Source: CAD feature listing. Evaluate the final solid. Frame: model axes, mm. A direction names the side the tool comes from. Give positions to 0.01 mm unless a question says otherwise; leave off trailing zeros. Order: outer loops, then holes, each group sorted by start corner. A loop starts at its lowest first (then second) coordinate and runs counter-clockwise, first axis right, second up. Notation, with made-up numbers: M 83,88.5 L 118,88.5 A12 ccw 118,101.5 Z; hole C 50.5,47.25 d10. An arc over 180 degrees is marked long. Use CSV: the item, a comma, the result in double quotes. Start each with the question number.
1. Pin query (flat end, axial travel): P1, Ø6, axis at x = 78, z = 2.5, coming from the +Y side; P2, Ø3, axis at x = -69, y = 5, coming from the +Z side; P3, Ø2, axis at x = 55.5, y = 2, coming from the +Z side. Return the tip coordinate at first contact, or that it passes through.
2. Section query A-A, the plane x = 77.5. Return the cut outline in (y, z), plus the area to 3 significant figures.
3. Line query: line 1 along Z through (x, y) = (65, 3.5); line 2 along X through (y, z) = (1.5, 4); line 3 along X through (y, z) = (1.5, -13.5). Output: solid intervals per line, ascending. Write a range as [from, to].
4. Section query B-B, the plane z = -67.5. Return the cut outline in (x, y).
5. Section query C-C, the plane y = 2. State how many separate pieces and enclosed holes the cut face has, plus the area to 3 significant figures.
6. Reachability of faces 5 (the flat face through (4, 10, -1)), 6 (the flat face through (33.887, 5, 8)), 7 (the flat face through (-80.901, 5, -85)), 8 (the cylindrical face through (76.395, 7.535, -7.936)), 9 (the flat face through (-80.901, 5, 85)) from +Z, -Z, +X, -X, +Y, -Y: full face, straight path, thin tool, end or side. Return the list, or none.
7. Mould query, pull axis Z, two halves, no side actions, for faces 1 (the flat face through (-65, 5, -80)), 2 (the flat face through (33.887, 5, -8)), 3 (the flat face through (-85, 5, 90)), 4 (the cylindrical face through (-43.254, 4.93, 88.662)). Classes: released by +Z, released by -Z, zero draft, split by the parting line, or undercut.
8. Section query D-D, the plane x = -72.5. Return the cut outline in (y, z), plus the area to 3 significant figures.
from build123d import *

# Parameters (mm, degrees)
BOSS_EXTRUDE1_DEPTH = 10
SKETCH2_R           = 1
SKETCH2_R_2         = 1.5
SKETCH2_W           = 33
SKETCH2_H           = 10
CUT_EXTRUDE2_DEPTH  = 15
SKETCH3_R           = 10
CUT_EXTRUDE3_DEPTH  = 5


with BuildPart() as part:
    # Sketch1 → Boss-Extrude1 (new body)
    with BuildSketch(Plane(origin=(0, 0, 0), x_dir=(1, 0, 0), z_dir=(0, 1, 0))):
        with BuildLine():
            Line((-89.389143795, -90), (-89.389143795, 90))
            Line((-89.389143795, 90), (10.610856205, 90))
            ThreePointArc((10.610856205, 90), (54.533138364, 81.496268076), (92.107774725, 57.214031174))
            ThreePointArc((92.107774725, 57.214031174), (94.381847518, 53.920998768), (95.182620993, 50))
            Line((95.182620993, 50), (95.182620993, -50))
            ThreePointArc((95.182620993, -50), (94.381847518, -53.920998768), (92.107774725, -57.214031174))
            ThreePointArc((92.107774725, -57.214031174), (54.533138364, -81.496268076), (10.610856205, -90))
            Line((10.610856205, -90), (-89.389143795, -90))
        make_face()
    extrude(amount=BOSS_EXTRUDE1_DEPTH)

    # Sketch2 → Cut-Extrude2 (cut, symmetric)
    with BuildSketch(Plane(origin=(0, 10, 0), x_dir=(1, 0, 0), z_dir=(0, 1, 0))):
        with Locations(Location((65, 14.131573434, 0), (0, 0, 90))):
            Circle(SKETCH2_R)
        with Locations(Location((27.688972694, 9.173126615, 0), (0, 0, 90))):
            Circle(SKETCH2_R_2)
        with Locations(Location((14.053243942, 9.173126615, 0), (0, 0, 90))):
            Circle(SKETCH2_R_2)
        with Locations(Location((14.053243942, -9.173126615, 0), (0, 0, 90))):
            Circle(SKETCH2_R_2)
        with Locations(Location((27.688972694, -9.173126615, 0), (0, 0, 90))):
            Circle(SKETCH2_R_2)
        with Locations(Location((65, -14.131573434, 0), (0, 0, 90))):
            Circle(SKETCH2_R)
        with BuildLine():
            Line((-40.968894473, 86.42714575), (-40.968894473, 80.97285425))
            ThreePointArc((-40.968894473, 80.97285425), (-43.204350858, 78.737397865), (-45.439807243, 80.97285425))
            Line((-45.439807243, 80.97285425), (-45.439807243, 86.42714575))
            ThreePointArc((-45.439807243, 86.42714575), (-43.204350858, 88.662602135), (-40.968894473, 86.42714575))
        make_face()
        with BuildLine():
            Line((38.845478036, 11.594873944), (38.845478036, 4.405126056))
            ThreePointArc((38.845478036, 4.405126056), (36.366254627, 1.925902647), (33.887031217, 4.405126056))
            Line((33.887031217, 4.405126056), (33.887031217, 11.594873944))
            ThreePointArc((33.887031217, 11.594873944), (36.366254627, 14.074097353), (38.845478036, 11.594873944))
        make_face()
        with Locations((-64.401012641, 85)):
            Rectangle(SKETCH2_W, SKETCH2_H)
        with BuildLine():
            Line((38.845478036, -11.594873944), (38.845478036, -4.405126056))
            ThreePointArc((38.845478036, -4.405126056), (36.366254627, -1.925902647), (33.887031217, -4.405126056))
            Line((33.887031217, -4.405126056), (33.887031217, -11.594873944))
            ThreePointArc((33.887031217, -11.594873944), (36.366254627, -14.074097353), (38.845478036, -11.594873944))
        make_face()
        with BuildLine():
            Line((-40.968894473, -86.42714575), (-40.968894473, -80.97285425))
            ThreePointArc((-40.968894473, -80.97285425), (-43.204350858, -78.737397865), (-45.439807243, -80.97285425))
            Line((-45.439807243, -80.97285425), (-45.439807243, -86.42714575))
            ThreePointArc((-45.439807243, -86.42714575), (-43.204350858, -88.662602135), (-40.968894473, -86.42714575))
        make_face()
        with Locations((-64.401012641, -85)):
            Rectangle(SKETCH2_W, SKETCH2_H)
    extrude(amount=CUT_EXTRUDE2_DEPTH, both=True, mode=Mode.SUBTRACT)

    # Sketch3 → Cut-Extrude3 (cut, symmetric)
    with BuildSketch(Plane(origin=(0, 10, 0), x_dir=(1, 0, 0), z_dir=(0, 1, 0))):
        with Locations(Location((82.479810043, 0, 0), (0, 0, 270))):
            Circle(SKETCH3_R)
    extrude(amount=CUT_EXTRUDE3_DEPTH, both=True, mode=Mode.SUBTRACT)


solid = part.part
Result set:
1,P1,"y = 5"
1,P2,"z = 80"
1,P3,"z = 81.51"
2,outline,"M 0,-69.14 L 10,-69.14 L 10,-8.67 L 5,-8.67 L 5,8.67 L 10,8.67 L 10,69.14 L 0,69.14 Z"
2,area,"1,300 mm2"
3,line 1,"[-76.68, -15.13], [-13.13, 13.13], [15.13, 76.68]"
3,line 2,"[-89.39, 33.92], [38.81, 95.18]"
3,line 3,"[-89.39, 34.78], [37.95, 64.22], [65.78, 95.18]"
4,outline,"M -89.39,0 L 79.82,0 L 79.82,10 L -89.39,10 Z"
5,separate pieces,"1"
5,enclosed holes,"10"
5,area,"30,500 mm2"
6,face 5,"+Z, -Z, +X, -X, +Y"
6,face 6,"+Y, -Y"
6,face 7,"-Z, +Y, -Y"
6,face 8,"+Y"
6,face 9,"+Z, +Y, -Y"
7,face 1,"released by -Z"
7,face 2,"undercut"
7,face 3,"released by +Z"
7,face 4,"undercut"
8,outline,"M 0,-80 L 10,-80 L 10,80 L 0,80 Z"
8,area,"1,600 mm2"
